Input: part model. Units: mm. Frame: model coordinates. Face numbers are marked on the shaded views. A direction names the side the tool comes from. Round coordinates to 2 decimals unless told otherwise and drop trailing zeros. Write each loop counter-clockwise with the first axis right and the second up, starting at its lowest first coordinate (ties: lowest second). Pieces come first, ordered by that corner, then holes. Notation, with made-up numbers: (29.25, 57) - (47.25, 57) arc R22 ccw to (47.25, 85) - close; hole circle Ø7 at (47, 31). An arc over 180 degrees is marked (long way). Use one line per item in the form item = value.
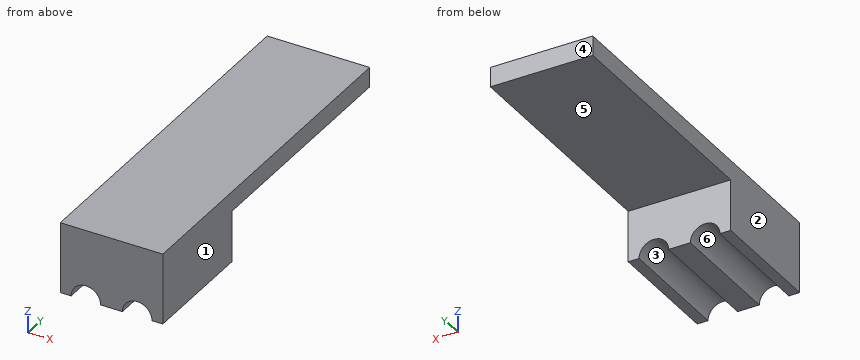
```python
from build123d import *

# Parameters (mm, degrees)
BOX016_W          = 30
BOX016_H          = 20
BOX016_DEPTH      = 9.2
BOX015_W          = 26
BOX015_H          = 12
BOX015_DEPTH      = 5.2
CYLINDER007_R     = 0.75
CYLINDER007_DEPTH = 7
ARRAY007_X_COUNT  = 2
ARRAY007_X_PITCH  = 2.6
ARRAY007_Y_COUNT  = 2
ARRAY007_Y_PITCH  = 1
BOX014_W          = 5.2
BOX014_H          = 18
BOX014_DEPTH      = 7.2


with BuildPart() as obj1:
    # Box016 → Box016 (new body)
    with BuildSketch(Plane(origin=(-1, -2, -5.6), x_dir=(1, 0, 0), z_dir=(0, 0, 1))):
        with Locations((15, 10)):
            Rectangle(BOX016_W, BOX016_H)
    extrude(amount=BOX016_DEPTH)


with BuildPart() as cube_10_base009:
    # Box015 → Box015 (new body)
    with BuildSketch(Plane(origin=(0, 6, 1), x_dir=(1, 0, 0), z_dir=(0, 0, 1))):
        with Locations((13, 6)):
            Rectangle(BOX015_W, BOX015_H)
    extrude(amount=BOX015_DEPTH)


with BuildPart() as array007:
    # Cylinder007 → Cylinder007 (new body)
    with BuildSketch(Plane(origin=(1.3, -1, 3.6), x_dir=(1, 0, 0), z_dir=(0, 1, 0))):
        Circle(CYLINDER007_R)
    extrude(amount=CYLINDER007_DEPTH)

    # Array007 X: Array007 ×2


with BuildPart() as array007_1:
    add(array007.part)
    with Locations(*[(i * ARRAY007_X_PITCH, 0, 0) for i in range(1, ARRAY007_X_COUNT)]):
        add(array007.part)

    # Array007 Y: Array007 ×2


with BuildPart() as array007_2:
    add(array007_1.part)
    with Locations(*[(0, i * ARRAY007_Y_PITCH, 0) for i in range(1, ARRAY007_Y_COUNT)]):
        add(array007_1.part)


with BuildPart() as obj2:
    # Box014 → Box014 (new body)
    with BuildSketch(Plane.XY):
        with Locations((2.6, 9)):
            Rectangle(BOX014_W, BOX014_H)
    extrude(amount=BOX014_DEPTH)

    # Cut015: cut Array007
    add(array007_2.part, mode=Mode.SUBTRACT)

    # Cut014: cut cube_10_base009
    add(cube_10_base009.part, mode=Mode.SUBTRACT)

    # Cut016: cut obj1
    add(obj1.part, mode=Mode.SUBTRACT)


solid = obj2.part
```
(1) Material intervals for L1, parallel to Y at x = 2.7, z = 6.15; L2, parallel to Z at x = 1.2, y = 7.5; L3, parallel to Z at x = 4.4, y = 2.25, sorted ascending.
Derived:
L1 = 0 to 6
L2 = 6.2 to 7.2
L3 = 4.16 to 7.2
(2) Access query for the marked faces 5 and 6. Directions: +Z, -Z, +X, -X, +Y, -Y. A direction counts if a zero-diameter tool reaches every point of the face in a straight line with its end or side. Return the directions, or none.
Derived:
face_5 = -Z, +X, -X, +Y
face_6 = -Z, +Y, -Y
(3) Cut plane A-A on x = 2.3. Output: boundary loops of the cut face in (y, z).
Derived:
outline = (0, 3.6) - (6, 3.6) - (6, 6.2) - (18, 6.2) - (18, 7.2) - (0, 7.2) - close
(4) Cut plane D-D on x = 3.9. Output: boundary loops of the cut face in (y, z).
Derived:
outline = (0, 4.35) - (6, 4.35) - (6, 6.2) - (18, 6.2) - (18, 7.2) - (0, 7.2) - close
(5) Cut plane B-B on y = 2. Output: boundary loops of the cut face in (x, z).
Derived:
outline = (0, 3.6) - (0.55, 3.6) arc R0.75 cw to (2.05, 3.6) - (3.15, 3.6) arc R0.75 cw to (4.65, 3.6) - (5.2, 3.6) - (5.2, 7.2) - (0, 7.2) - close
(6) Cut plane C-C on z = 5.9. Output: boundary loops of the cut face in (x, y).
Derived:
outline = (0, 0) - (5.2, 0) - (5.2, 6) - (0, 6) - close
(7) Draft query along X for the marked faces 1, 2, 3 and 4. Return one class per face: released by +X, released by -X, zero draft, split by the parting line, or undercut.
Derived:
face_1 = released by +X
face_2 = released by -X
face_3 = undercut
face_4 = zero draft
(8) First-contact query: pin 1 Ø1.6 at (x, y) = (3, 10) entering from -Z; pin 2 Ø2 at (x, z) = (1.5, 5) entering from +Y. Flat tips, straight axial feed; report the tip coordinate or a pass-through.
Derived:
pin_1 = 6.2
pin_2 = 6
